```python
from build123d import *

# Parameters (mm, degrees)
F1_DEPTH = 784.225
F2_R     = 1.5875
F3_R     = 0.635


with BuildPart() as f1:
    # F0 (on Front) → F1 (new body, symmetric)
    with BuildSketch(Plane.XZ):
        with BuildLine():
            Line((0, 37.3126), (0, 0))
            Line((0, 0), (41.275, 0))
            Line((41.275, 0), (41.275, 37.3126))
            ThreePointArc((41.275, 37.3126), (37.3126, 41.275), (33.3502, 37.3126))
            Line((33.3502, 37.3126), (34.9377, 37.3126))
            ThreePointArc((34.9377, 37.3126), (37.3126, 39.6875), (39.6875, 37.3126))
            Line((39.6875, 37.3126), (39.6875, 1.5875))
            Line((39.6875, 1.5875), (1.5875, 1.5875))
            Line((1.5875, 1.5875), (1.5875, 37.3126))
            ThreePointArc((1.5875, 37.3126), (3.9624, 39.6875), (6.3373, 37.3126))
            Line((6.3373, 37.3126), (7.9248, 37.3126))
            ThreePointArc((7.9248, 37.3126), (3.9624, 41.275), (0, 37.3126))
        make_face()
    extrude(amount=F1_DEPTH, both=True)

    # F2
    f2_edges = [f1.edges().sort_by_distance(p)[0] for p in [
        (0, 0, 0),
        (41.275, 0, 0),
        (1.5875, 0, 1.5875),
        (39.6875, 0, 1.5875),
    ]]
    fillet(f2_edges, radius=F2_R)

    # F3
    f3_edges = [f1.edges().sort_by_distance(p)[0] for p in [
        (6.3373, 0, 37.3126),
        (7.9248, 0, 37.3126),
        (33.3502, 0, 37.3126),
        (34.9377, 0, 37.3126),
    ]]
    fillet(f3_edges, radius=F3_R)


solid = f1.part
```
Source: CAD feature listing. Evaluate the final solid. Frame: model axes, mm. A direction names the side the tool comes from. Coordinates: 2 decimals unless noted, no trailing zeros. Write each loop counter-clockwise with the first axis right and the second up, starting at its lowest first coordinate (ties: lowest second). Pieces come first, ordered by that corner, then holes. Notation, with made-up numbers: M 61,-11.5 L 103,-11.5 A24 ccw 103,2.5 Z; hole C 34.25,4 d10. An arc over 180 degrees is marked long. Answer as a JSON object with one key per item and string values.
1. Cut plane C-C on x = 15.5. Output: boundary loops of the cut face in (y, z) (1 decimal).
Evaluation:
{"outline": "M -784.2,0 L 784.2,0 L 784.2,1.6 L -784.2,1.6 Z"}
2. Ray query, L1, parallel to X at y = -249, z = 37.5; L2, parallel to Z at x = 34, y = 26; L3, parallel to X at y = 131, z = 7.5 (1 decimal). Return the intervals inside material, ascending.
Evaluation:
{"L1": "0 to 1.59, 6.45 to 7.68, 33.6 to 34.82, 39.68 to 41.27", "L2": "0 to 1.59, 37.31 to 39.49", "L3": "0 to 1.6, 39.7 to 41.3"}
3. Access query for faces 4 (the flat face through (21, -11, 1.588)), 5 (the flat face through (20, -11, 0)). Directions: +Z, -Z, +X, -X, +Y, -Y. A direction counts if a zero-diameter tool reaches every point of the face in a straight line with its end or side. Return the directions, or none.
Evaluation:
{"face 4": "+Y, -Y", "face 5": "-Z, +X, -X, +Y, -Y"}
4. Draft query along X for faces 1 (the flat face through (21, 784.225, 1)), 2 (the flat face through (0, -11, 20)), 3 (the flat face through (1.588, -11, 20)). Return one class per face: released by +X, released by -X, zero draft, split by the parting line, or undercut.
Evaluation:
{"face 1": "zero draft", "face 2": "released by -X", "face 3": "undercut"}
5. Cut plane A-A on z = 27. Output: boundary loops of the cut face in (x, y) (1 decimal).
Evaluation:
{"outline": "M 0,-784.2 L 1.6,-784.2 L 1.6,784.2 L 0,784.2 Z; M 39.7,-784.2 L 41.3,-784.2 L 41.3,784.2 L 39.7,784.2 Z"}
6. Contact query for flat-ended pins moving along their axis: P1, Ø4, axis at x = 32.5, y = -380.5, coming from the +Z side; P2, Ø10, axis at x = 9.5, z = 18, coming from the -Y side. Output: stop coordinate, or through.
Evaluation:
{"P1": "z = 40.1", "P2": "through"}
